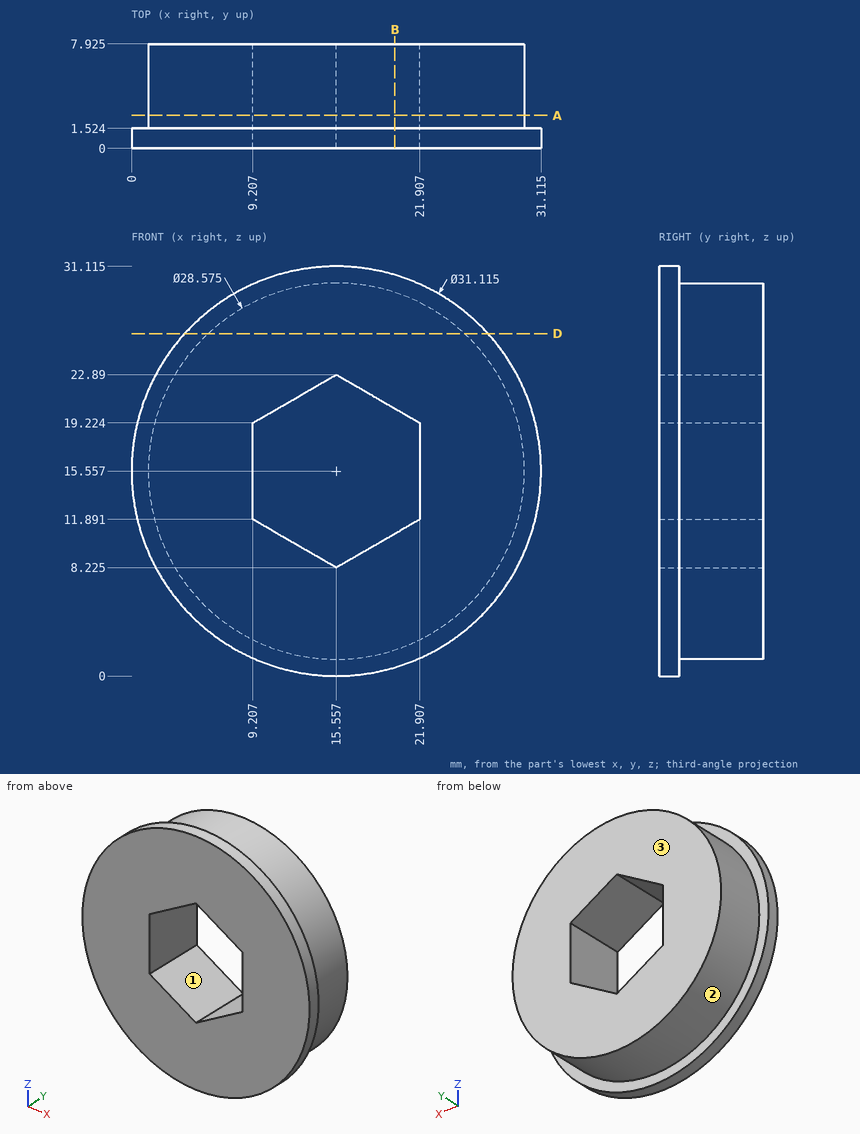
Input: dimensioned drawing with shaded views. Units: mm. Origin: part minimum x, y, z. A direction names the side the tool comes from. Give positions to 0.01 mm unless a question says otherwise; leave off trailing zeros. Write each loop counter-clockwise with the first axis right and the second up, starting at its lowest first coordinate (ties: lowest second). Pieces come first, ordered by that corner, then holes. Notation, with made-up numbers: (29.25, 88.5) - (72.25, 88.5) arc R27 ccw to (72.25, 121.5) - close; hole circle Ø6 at (74.5, 1.5). An arc over 180 degrees is marked (long way). Write item = value, one per line. Start each with the question number.
1) Pin query (flat end, axial travel): pin 1 (1 mm diameter, centred on x = 7.5, y = 6, fed in from -Z); pin 2 (2 mm diameter, centred on y = 3, z = 16.5, fed in from -X). Return the tip coordinate at first contact, or that it passes through.
2) Material intervals for L1, parallel to X at y = 1, z = 18.5 (1 decimal); L2, parallel to Z at x = 11.5, y = 3 (1 decimal); L3, parallel to X at y = 5.75, z = 17, sorted ascending. Write a range as [from, to].
3) Cut plane A-A (y = 2.5). Return loops of the section in (x, z) (1 decimal).
4) Cut plane B-B (x = 20). Return loops of the section in (y, z) (1 decimal), and give its area (3 significant figures).
5) Reachability of the marked faces 1, 2 and 3 from +Z, -Z, +X, -X, +Y, -Y: full face, straight path, thin tool, end or side. Return the list, or none.
6) Cut plane D-D (z = 26). Return loops of the section in (x, y) (1 decimal).
Answers follow:
q1.pin_1 = 3.43
q1.pin_2 = 1.27
q2.L1 = [0.3, 9.2], [21.9, 30.8]
q2.L2 = [1.9, 10.6], [20.5, 29.3]
q2.L3 = [1.34, 9.21], [21.91, 29.77]
q3.outline = circle Ø28.6 at (15.6, 15.6); hole (9.2, 11.9) - (15.6, 8.2) - (21.9, 11.9) - (21.9, 19.2) - (15.6, 22.9) - (9.2, 19.2) - close
q4.outline = (0, 0.6) - (1.5, 0.6) - (1.5, 2) - (7.9, 2) - (7.9, 10.8) - (0, 10.8) - close; (0, 20.3) - (7.9, 20.3) - (7.9, 29.1) - (1.5, 29.1) - (1.5, 30.5) - (0, 30.5) - close
q4.area = 144 mm^2
q5.face_1 = +Y, -Y
q5.face_2 = +Y
q5.face_3 = +Z, -Z, +X, -X, +Y
q6.outline = (4, 0) - (27.1, 0) - (27.1, 1.5) - (25.3, 1.5) - (25.3, 7.9) - (5.8, 7.9) - (5.8, 1.5) - (4, 1.5) - close
